Could you check a few things on this model? Use its own coordinates, in mm. A direction names the side the tool comes from. Give positions to 0.01 mm unless a question says otherwise; leave off trailing zeros. Order: outer loops, then holes, each group sorted by start corner. A loop starts at its lowest first (then second) coordinate and runs counter-clockwise, first axis right, second up.
(1) Imagine slicing it at B-B, the plane z = 2.25. Write out the boundary of the cut face in (x, y), then the cut area to 3 significant figures.
(2) If we mould it in two halves opening along Z, with no side actions, what happens to faces 1 (the flat face through (-1, 3, 21.844)), 2 (the cylindrical face through (-2.93, 5.634, 21.2)), 3 (the cylindrical face through (-1.266, -5.703, 19.93))? For each: released by +Z, released by -Z, zero draft, split by the parting line, or undercut.
(3) Imagine slicing it at C-C, the plane x = -2.25. Write out the boundary of the cut face in (y, z), then the cut area to 3 significant figures.
(4) If I drill on probe 1 along Z at (x, y) = (6.25, -0.75); probe 2 along Z at (x, y) = (-4.25, -5.75); probe 3 along X at (y, z) = (-2.5, 13.5), over which ranges is the centre line in solid material (lowest first)?
(5) Imagine slicing it at D-D, the plane x = -5.5. Write out the boundary of the cut face in (y, z).
(6) Will these pins go through, and if not, where does the flat tip stop? pin 1 (1.5 mm diameter, centred on x = -1, y = 2.5, fed in from -Z); pin 2 (8 mm diameter, centred on y = 0.5, z = 11.5, fed in from +X); pin 3 (2 mm diameter, centred on x = 4.5, z = 11, fed in from -Y); pin 4 (1 mm diameter, centred on y = -5.5, z = 4.5, fed in from +X).
(7) Imagine slicing it at A-A, the plane y = 0. Write out the boundary of the cut face in (x, z).
(8) On a 3-axis mill with a long thin cutter (end or side, diameter ignored), from which of +Z, -Z, +X, -X, +Y, -Y can I reach the whole of each face in a straight line? I mean faces 4 (the flat face through (6.35, 0, 10)), 5 (the flat face through (-6.35, 0, 10)), 6 (the flat face through (3.219, 5.474, 10.161)). Say none if no direction works.
from build123d import *

# Parameters (mm, degrees)
BOSS_EXTRU_1_DEPTH      = 19.304
ESQUISSE2_R             = 7.62
BOSS_EXTRU_2_DEPTH      = 1.27
ESQUISSE3_R             = 5.842
BOSS_EXTRU_3_DEPTH      = 1.27
ESQUISSE4_R             = 6.35
BOSS_EXTRU_4_DEPTH      = 1.27
ESQUISSE5_R             = 3
ENL_V_MAT_EXTRU_1_DEPTH = 25.357527297


with BuildPart() as part:
    # Esquisse1 → Boss.-Extru.1 (new body)
    with BuildSketch(Plane.XY):
        Polygon((0, 7.332348419), (-6.35, 3.666174209), (-6.35, -3.666174209), (0, -7.332348419), (6.35, -3.666174209), (6.35, 3.666174209), align=None)
    extrude(amount=BOSS_EXTRU_1_DEPTH)

    # Esquisse2 → Boss.-Extru.2 (add)
    with BuildSketch(Plane.XY):
        Circle(ESQUISSE2_R)
    extrude(amount=BOSS_EXTRU_2_DEPTH)

    # Esquisse3 → Boss.-Extru.3 (add)
    with BuildSketch(Plane.XY.offset(19.304)):
        Circle(ESQUISSE3_R)
    extrude(amount=BOSS_EXTRU_3_DEPTH)

    # Esquisse4 → Boss.-Extru.4 (add)
    with BuildSketch(Plane.XY.offset(20.574)):
        with Locations(Location((0, 0, 0), (0, 0, 180))):
            Circle(ESQUISSE4_R)
    extrude(amount=BOSS_EXTRU_4_DEPTH)

    # Esquisse5 → Enlèv. mat.-Extru.1 (cut, through all)
    with BuildSketch(Plane.XY):
        Circle(ESQUISSE5_R)
    extrude(amount=ENL_V_MAT_EXTRU_1_DEPTH, mode=Mode.SUBTRACT)


solid = part.part
Answer block:
1. outline: (-6.35, -3.67) - (0, -7.33) - (6.35, -3.67) - (6.35, 3.67) - (0, 7.33) - (-6.35, 3.67) - close; hole circle Ø6 at (0, 0)
1. area: 111 mm2
2. face 1: released by +Z
2. face 2: zero draft
2. face 3: undercut
3. outline: (-7.28, 0) - (-1.98, 0) - (-1.98, 21.84) - (-5.94, 21.84) - (-5.94, 20.57) - (-5.39, 20.57) - (-5.39, 19.3) - (-6.03, 19.3) - (-6.03, 1.27) - (-7.28, 1.27) - close; (1.98, 0) - (7.28, 0) - (7.28, 1.27) - (6.03, 1.27) - (6.03, 19.3) - (5.39, 19.3) - (5.39, 20.57) - (5.94, 20.57) - (5.94, 21.84) - (1.98, 21.84) - close
3. area: 178 mm2
4. probe 1: z = 0 to 19.3, 20.57 to 21.84
4. probe 2: z = 0 to 1.27
4. probe 3: x = -6.35 to -1.66, 1.66 to 6.35
5. outline: (-5.27, 0) - (5.27, 0) - (5.27, 1.27) - (4.16, 1.27) - (4.16, 19.3) - (1.97, 19.3) - (1.97, 20.57) - (3.17, 20.57) - (3.17, 21.84) - (-3.17, 21.84) - (-3.17, 20.57) - (-1.97, 20.57) - (-1.97, 19.3) - (-4.16, 19.3) - (-4.16, 1.27) - (-5.27, 1.27) - close
6. pin 1: stops at z = 0
6. pin 2: stops at x = 6.35
6. pin 3: stops at y = -5.31
6. pin 4: stops at x = 4.04
7. outline: (-7.62, 0) - (-3, 0) - (-3, 21.84) - (-6.35, 21.84) - (-6.35, 20.57) - (-5.84, 20.57) - (-5.84, 19.3) - (-6.35, 19.3) - (-6.35, 1.27) - (-7.62, 1.27) - close; (3, 0) - (7.62, 0) - (7.62, 1.27) - (6.35, 1.27) - (6.35, 19.3) - (5.84, 19.3) - (5.84, 20.57) - (6.35, 20.57) - (6.35, 21.84) - (3, 21.84) - close
8. face 4: +Z, +X, +Y, -Y
8. face 5: +Z, -X, +Y, -Y
8. face 6: +Z, +X, +Y
